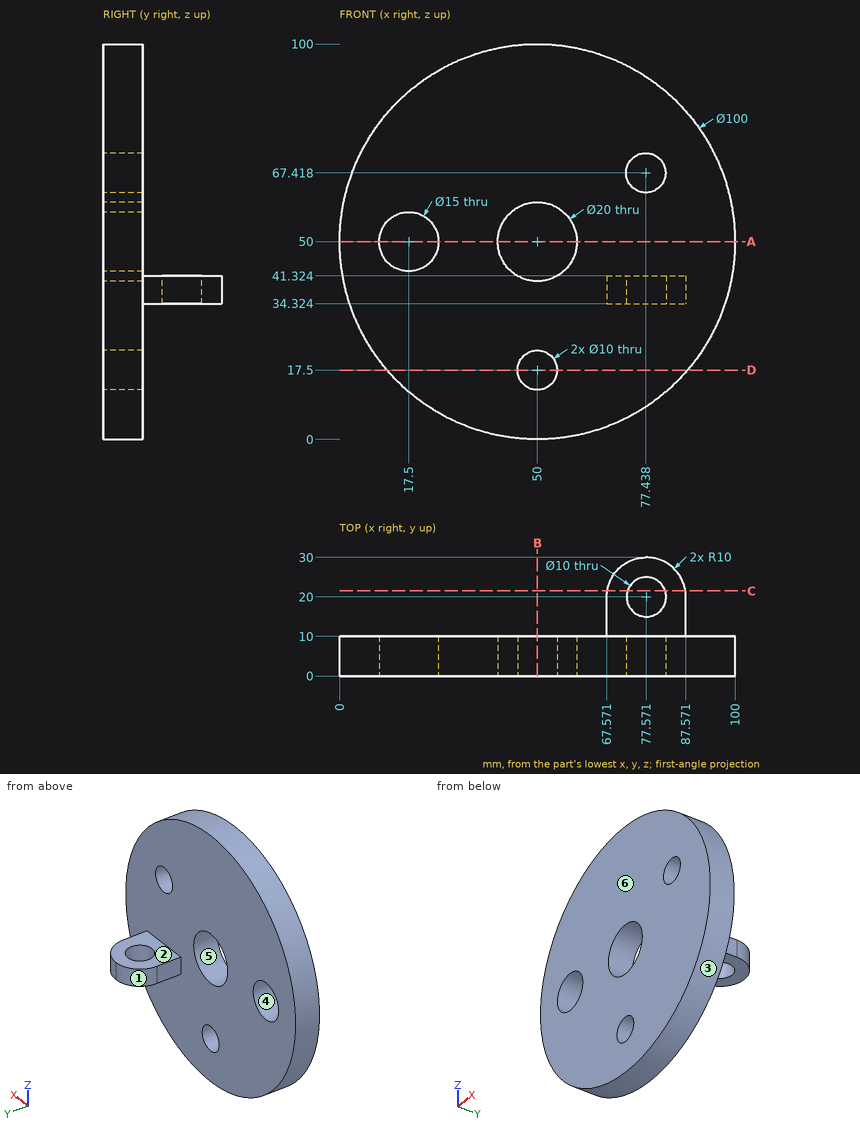
Here's the drawing with two shaded views (mm, measured from the low corner). I have some questions. A direction names the side the tool comes from. Give positions to 0.01 mm unless a question says otherwise; leave off trailing zeros. Write each loop counter-clockwise with the first axis right and the second up, starting at its lowest first coordinate (ties: lowest second). Pieces come first, ordered by that corner, then holes. Notation, with made-up numbers: (87, 27.25) -> (128, 27.25) arc R28 ccw to (128, 63.25) -> close; hole circle Ø5 at (39.25, 1). An arc over 180 degrees is marked (long way). Answer as a JSON object with one key per item and string values. Group by question number.
Item 1: Suppose I cut it at C-C (y = 21.5). Please give me the cut outline in (x, z).
Item 2: For the marked faces 1 and 2, which set-ups out of +Z, -Z, +X, -X, +Y, -Y let a thin tool reach every point of the face, with its end or its side?
Item 3: Suppose I cut it at B-B (x = 50). Please give me the cut outline in (y, z), plus the area to 3 significant figures.
Item 4: Please list where these lines run through material, in increasing order: line 1 (X direction, y = 3.25, z = 50); line 2 (Y direction, x = 64, z = 12.5); line 3 (Z direction, x = 81.5, y = 4) (1 decimal). Write a range as [from, to].
Item 5: Suppose I cut it at A-A (z = 50). Please give me the cut outline in (x, y), plus the area to 3 significant figures.
Item 6: I'm going to push flat-ended pins straight in: P1, Ø10, axis at x = 72.5, y = 24.5, coming from the -Z side; P2, Ø7.5, axis at y = 12.5, z = 36, coming from the -X side; P3, Ø13, axis at x = 77.44, z = 67.42, coming from the +Y side. Where does each tip first touch, or does it pass through?
Item 7: Suppose I cut it at D-D (z = 17.5). Please give me the cut outline in (x, y), plus the area to 3 significant figures.
Item 8: We'd pull the mould along X, two halves only. Please class the marked faces 3, 4, 5 and 6: +X half, -X half, draft (parallel to the pull), parting line (faces both ways), or undercut.
Findings:
{
 "1": {"outline": "(67.68, 34.32) -> (72.8, 34.32) -> (72.8, 41.32) -> (67.68, 41.32) -> close; (82.34, 34.32) -> (87.46, 34.32) -> (87.46, 41.32) -> (82.34, 41.32) -> close"},
 "2": {"face 1": "+Z, -Z, -X, +Y", "face 2": "+Z, +X, -X, +Y"},
 "3": {"outline": "(0, 0) -> (10, 0) -> (10, 12.5) -> (0, 12.5) -> close; (0, 22.5) -> (10, 22.5) -> (10, 40) -> (0, 40) -> close; (0, 60) -> (10, 60) -> (10, 100) -> (0, 100) -> close", "area": "700 mm²"},
 "4": {"line 1": "x = [0, 10], [25, 40], [60, 100]", "line 2": "y = [0, 10]", "line 3": "z = [11.2, 64.5], [70.3, 88.8]"},
 "5": {"outline": "(0, 0) -> (10, 0) -> (10, 10) -> (0, 10) -> close; (25, 0) -> (40, 0) -> (40, 10) -> (25, 10) -> close; (60, 0) -> (100, 0) -> (100, 10) -> (60, 10) -> close", "area": "650 mm²"},
 "6": {"P1": "stops at z = 34.32", "P2": "stops at x = 1.27", "P3": "stops at y = 10"},
 "7": {"outline": "(12, 0) -> (45, 0) -> (45, 10) -> (12, 10) -> close; (55, 0) -> (88, 0) -> (88, 10) -> (55, 10) -> close", "area": "660 mm²"},
 "8": {"face 3": "parting line", "face 4": "undercut", "face 5": "undercut", "face 6": "draft"}
}
